For this review, take the finished solid that the model builds, in its own axes (mm). A direction names the side the tool comes from. Round coordinates to 2 decimals unless told otherwise and drop trailing zeros. Order: outer loops, then holes, each group sorted by start corner. A loop starts at its lowest first (then second) coordinate and runs counter-clockwise, first axis right, second up. Notation, with made-up numbers: (32.5, 86) -> (39.5, 86) arc R22 cw to (39.5, 115) -> close; hole circle Ø5 at (44, -27.5). An arc over 180 degrees is marked (long way). Answer in a Markdown table with one row per item.
```python
from build123d import *

# Parameters (mm, degrees)
CORTE_EXTERIOR_R        = 3.500001168
SALIENTE_EXTRUIR1_DEPTH = 3
CORTAR_EXTRUIR1_DEPTH   = 1
CORTAR_EXTRUIR2_DEPTH   = 0.1


with BuildPart() as part:
    # Corte exterior → Saliente-Extruir1 (new body)
    with BuildSketch(Plane.XY):
        with BuildLine():
            Line((19.521996462, -6.085833738), (11.021996462, -6.085833738))
            ThreePointArc((11.021996462, -6.085833738), (7.486462556, -7.550299832), (6.021996462, -11.085833738))
            Line((6.021996462, -11.085833738), (6.021996462, -21.085833738))
            ThreePointArc((6.021996462, -21.085833738), (7.486462556, -24.621367644), (11.021996462, -26.085833738))
            Line((11.021996462, -26.085833738), (55.021996462, -26.085833738))
            ThreePointArc((55.021996462, -26.085833738), (58.557530368, -24.621367644), (60.021996462, -21.085833738))
            Line((60.021996462, -21.085833738), (60.021996462, -11.085833738))
            ThreePointArc((60.021996462, -11.085833738), (58.557530368, -7.550299832), (55.021996462, -6.085833738))
            Line((55.021996462, -6.085833738), (46.514841363, -6.085833738))
            Line((46.514841363, -6.085833738), (46.521996462, 58.812041738))
            ThreePointArc((46.521996462, 58.812041738), (45.350423587, 61.640468863), (42.521996462, 62.812041738))
            Line((42.521996462, 62.812041738), (23.521996462, 62.812041738))
            ThreePointArc((23.521996462, 62.812041738), (20.693569337, 61.640468863), (19.521996462, 58.812041738))
            Line((19.521996462, 58.812041738), (19.521996462, -6.085833738))
        make_face()
        with Locations((33.021996462, 7.812041474)):
            Circle(CORTE_EXTERIOR_R, mode=Mode.SUBTRACT)
        with BuildLine():
            Line((55.29494797, -12.330366391), (52.77320204, -10.049840692))
            ThreePointArc((52.77320204, -10.049840692), (33.021996462, -18.817961696), (13.270789317, -10.049842109))
            Line((13.270789317, -10.049842109), (10.749043386, -12.330367808))
            ThreePointArc((10.749043386, -12.330367808), (33.021996462, -22.217961696), (55.29494797, -12.330366391))
        make_face(mode=Mode.SUBTRACT)
    extrude(amount=SALIENTE_EXTRUIR1_DEPTH)

    # Grabado Superficie → Cortar-Extruir1 (cut)
    with BuildSketch(Plane.XY):
        with BuildLine():
            Line((35.89134848, 9.816243852), (35.017032688, 22.202862127))
            ThreePointArc((35.017032688, 22.202862127), (33.021996462, 24.062041474), (31.026960236, 22.202862127))
            Line((31.026960236, 22.202862127), (30.152644444, 9.816243852))
            ThreePointArc((30.152644444, 9.816243852), (33.021996462, 11.312042642), (35.89134848, 9.816243852))
        make_face()
    extrude(amount=CORTAR_EXTRUIR1_DEPTH, mode=Mode.SUBTRACT)

    # grabado linea medio → Cortar-Extruir2 (cut)
    with BuildSketch(Plane.XY):
        Polygon((23.601996462, 43.022041738), (19.521996462, 43.022041738), (19.521996462, 58.172041738), (27.661996462, 58.172041738), (27.661996462, 62.812041738), (30.181996462, 62.812041738), (30.181996462, 58.170825238), (46.521996462, 57.970825238), (46.521996462, 34.942041738), (30.181996462, 34.942041738), (30.181996462, 30.302041738), (27.661996462, 30.302041738), (27.661996462, 34.942041738), (23.601996462, 34.942041738), align=None)
    extrude(amount=CORTAR_EXTRUIR2_DEPTH, mode=Mode.SUBTRACT)


solid = part.part
```
Q1. Tool access review of faces 1 (the face through (33, 17, 1)), 2 (the face through (15, -6.086, 1)), 3 (the face through (54.052, -11.206, 1.479)), 4 (the face through (33, -26.086, 1)): name each direction out of +Z, -Z, +X, -X, +Y, -Y from which nothing blocks a thin tool from reaching the whole face with its end or side.
Answer key:
| item | result |
|---|---|
| face 1 | -Z |
| face 2 | +Z, -Z, -X, +Y |
| face 3 | +Z, -Z |
| face 4 | +Z, -Z, +X, -X, -Y |
Q2. Clearance check with flat-ended pins moving along their axes: pin 1 Ø1.5 at (y, z) = (49.5, 1) entering from +X; pin 2 Ø0.9 at (y, z) = (38.5, 2) entering from -X; pin 3 Ø1.5 at (x, z) = (51, 1.5) entering from +Y. State where each tip first meets the part, or that it passes through.
Answer key:
| item | result |
|---|---|
| pin 1 | stops at x = 46.52 |
| pin 2 | stops at x = 19.52 |
| pin 3 | stops at y = -6.09 |
Q3. Take a section at B-B, the plane x = 34. Write out the cut boundary in (y, z), then the cut area to 3 significant figures.
Answer key:
| item | result |
|---|---|
| outline | (-26.09, 0) -> (-22.2, 0) -> (-22.2, 3) -> (-26.09, 3) -> close; (-18.8, 0) -> (4.45, 0) -> (4.45, 3) -> (-18.8, 3) -> close; (11.17, 1) -> (23.81, 1) -> (23.81, 0) -> (34.94, 0) -> (34.94, 0.1) -> (58.12, 0.1) -> (58.12, 0) -> (62.81, 0) -> (62.81, 3) -> (11.17, 3) -> close |
| area | 221 mm^2 |
Q4. The part is to be moulded in two halves that separate along X. For faces 5 (the face through (7.53, -7.51, 1.48)), 6 (the face through (38, 60, 0)), 7 (the face through (32.263, 4.395, 1.479)), say which applies: +X half, -X half, draft (parallel to the pull), parting line (faces both ways), or undercut.
Answer key:
| item | result |
|---|---|
| face 5 | -X half |
| face 6 | draft |
| face 7 | undercut |
Q5. Take a section at D-D, the plane y = 39.5. Write out the cut boundary in (x, z).
Answer key:
| item | result |
|---|---|
| outline | (19.52, 0) -> (23.6, 0) -> (23.6, 0.1) -> (46.52, 0.1) -> (46.52, 3) -> (19.52, 3) -> close |
Q6. To check wall thickness, follow probe 1 along X at (y, z) = (16, 2.65); probe 2 along Y at (x, z) = (41.5, 1.6); probe 3 along Y at (x, z) = (21, 2). State the ranges of each line that lie inside material, in increasing order.
Answer key:
| item | result |
|---|---|
| probe 1 | x = 19.52 to 46.52 |
| probe 2 | y = -26.09 to -21, -17.43 to 62.81 |
| probe 3 | y = -26.09 to -19.71, -15.95 to 61.92 |
Q7. Take a section at C-C, the plane z = 2. Write out the cut boundary in (x, y), then the cut area to 3 significant figures.
Answer key:
| item | result |
|---|---|
| outline | (6.02, -21.09) arc R5 ccw to (11.02, -26.09) -> (55.02, -26.09) arc R5 ccw to (60.02, -21.09) -> (60.02, -11.09) arc R5 ccw to (55.02, -6.09) -> (46.51, -6.09) -> (46.52, 58.81) arc R4 ccw to (42.52, 62.81) -> (23.52, 62.81) arc R4 ccw to (19.52, 58.81) -> (19.52, -6.09) -> (11.02, -6.09) arc R5 ccw to (6.02, -11.09) -> close; hole (10.75, -12.33) arc R30.03 ccw to (55.29, -12.33) -> (52.77, -10.05) arc R26.63 cw to (13.27, -10.05) -> close; hole circle Ø7 at (33.02, 7.81) |
| area | 2,710 mm^2 |
Q8. Take a section at A-A, the plane x = 17.5. Write out the cut boundary in (y, z).
Answer key:
| item | result |
|---|---|
| outline | (-26.09, 0) -> (-17.9, 0) -> (-17.9, 3) -> (-26.09, 3) -> close; (-13.83, 0) -> (-6.09, 0) -> (-6.09, 3) -> (-13.83, 3) -> close |
